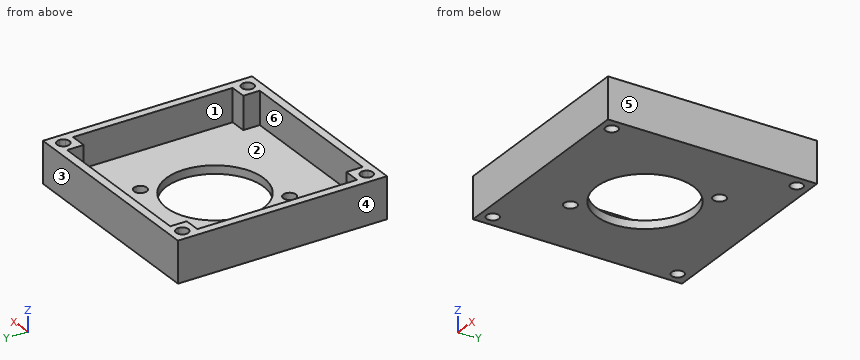
```python
from build123d import *
from build123d.topology import SkipClean

# Parameters (mm, degrees)
SKETCH3_W           = 50.8
SKETCH3_H           = 50.8
SKETCH3_R           = 11.8
SKETCH3_R_2         = 1.55
BOSS_EXTRUDE5_DEPTH = 2
SKETCH1_W           = 2
SKETCH1_H           = 38.8
SKETCH1_W_2         = 38.8
SKETCH1_H_2         = 2
BOSS_EXTRUDE6_DEPTH = 10
SKETCH7_R           = 1.5
CUT_EXTRUDE2_DEPTH  = 37.80108694


with BuildPart() as part:
    # Sketch3 → Boss-Extrude5 (new body)
    with BuildSketch(Plane.XY):
        Rectangle(SKETCH3_W, SKETCH3_H)
        Circle(SKETCH3_R, mode=Mode.SUBTRACT)
        with Locations((-9.5, -12)):
            Circle(SKETCH3_R_2, mode=Mode.SUBTRACT)
        with Locations((9.5, 12)):
            Circle(SKETCH3_R_2, mode=Mode.SUBTRACT)
    extrude(amount=BOSS_EXTRUDE5_DEPTH)

    # Sketch1 → Boss-Extrude6 (add)
    with BuildSketch(Plane.XY):
        with Locations((24.4, 0)):
            Rectangle(SKETCH1_W, SKETCH1_H)
        with BuildLine():
            Line((21.281966011, -23.4), (19.4, -23.4))
            Line((19.4, -23.4), (19.4, -25.4))
            Line((19.4, -25.4), (25.4, -25.4))
            Line((25.4, -25.4), (25.4, -19.4))
            Line((25.4, -19.4), (23.4, -19.4))
            Line((23.4, -19.4), (23.4, -21.281966011))
            ThreePointArc((23.4, -21.281966011), (23.769306394, -21.787627564), (23.9, -22.4))
            ThreePointArc((23.9, -22.4), (22.935233135, -23.801258538), (21.281966011, -23.4))
        make_face()
        with BuildLine():
            Line((19.4, -19.4), (19.4, -23.4))
            Line((19.4, -23.4), (21.281966011, -23.4))
            ThreePointArc((21.281966011, -23.4), (21.339339828, -21.339339828), (23.4, -21.281966011))
            Line((23.4, -21.281966011), (23.4, -19.4))
            Line((23.4, -19.4), (19.4, -19.4))
        make_face()
        with Locations((0, -24.4)):
            Rectangle(SKETCH1_W_2, SKETCH1_H_2)
        with BuildLine():
            ThreePointArc((-20.9, -22.4), (-20.998741462, -22.935233135), (-21.281966011, -23.4))
            Line((-21.281966011, -23.4), (-19.4, -23.4))
            Line((-19.4, -23.4), (-19.4, -19.4))
            Line((-19.4, -19.4), (-23.4, -19.4))
            Line((-23.4, -19.4), (-23.4, -21.281966011))
            ThreePointArc((-23.4, -21.281966011), (-21.787627564, -21.030693606), (-20.9, -22.4))
        make_face()
        with BuildLine():
            Line((-19.4, -23.4), (-21.281966011, -23.4))
            ThreePointArc((-21.281966011, -23.4), (-23.460660172, -23.460660172), (-23.4, -21.281966011))
            Line((-23.4, -21.281966011), (-23.4, -19.4))
            Line((-23.4, -19.4), (-25.4, -19.4))
            Line((-25.4, -19.4), (-25.4, -25.4))
            Line((-25.4, -25.4), (-19.4, -25.4))
            Line((-19.4, -25.4), (-19.4, -23.4))
        make_face()
        with Locations((-24.4, 0)):
            Rectangle(SKETCH1_W, SKETCH1_H)
        with BuildLine():
            Line((-25.4, 19.4), (-23.4, 19.4))
            Line((-23.4, 19.4), (-23.4, 21.281966011))
            ThreePointArc((-23.4, 21.281966011), (-23.460660172, 23.460660172), (-21.281966011, 23.4))
            Line((-21.281966011, 23.4), (-19.4, 23.4))
            Line((-19.4, 23.4), (-19.4, 25.4))
            Line((-19.4, 25.4), (-25.4, 25.4))
            Line((-25.4, 25.4), (-25.4, 19.4))
        make_face()
        with BuildLine():
            Line((-23.4, 21.281966011), (-23.4, 19.4))
            Line((-23.4, 19.4), (-19.4, 19.4))
            Line((-19.4, 19.4), (-19.4, 23.4))
            Line((-19.4, 23.4), (-21.281966011, 23.4))
            ThreePointArc((-21.281966011, 23.4), (-20.998741462, 22.935233135), (-20.9, 22.4))
            ThreePointArc((-20.9, 22.4), (-21.787627564, 21.030693606), (-23.4, 21.281966011))
        make_face()
        with Locations((0, 24.4)):
            Rectangle(SKETCH1_W_2, SKETCH1_H_2)
        with BuildLine():
            Line((23.4, 21.281966011), (23.4, 19.4))
            Line((23.4, 19.4), (25.4, 19.4))
            Line((25.4, 19.4), (25.4, 25.4))
            Line((25.4, 25.4), (19.4, 25.4))
            Line((19.4, 25.4), (19.4, 23.4))
            Line((19.4, 23.4), (21.281966011, 23.4))
            ThreePointArc((21.281966011, 23.4), (22.935233135, 23.801258538), (23.9, 22.4))
            ThreePointArc((23.9, 22.4), (23.769306394, 21.787627564), (23.4, 21.281966011))
        make_face()
        with BuildLine():
            Line((19.4, 19.4), (23.4, 19.4))
            Line((23.4, 19.4), (23.4, 21.281966011))
            ThreePointArc((23.4, 21.281966011), (21.339339828, 21.339339828), (21.281966011, 23.4))
            Line((21.281966011, 23.4), (19.4, 23.4))
            Line((19.4, 23.4), (19.4, 19.4))
        make_face()
    extrude(amount=BOSS_EXTRUDE6_DEPTH)

    # Sketch7 → Cut-Extrude2 (cut, through all)
    with SkipClean():  # the faces are left unmerged after this step: merging them gives an invalid solid
        with BuildSketch(Plane.XY.offset(2)):
            with Locations((-22.4, 22.4)):
                Circle(SKETCH7_R)
            with Locations(Location((22.4, 22.4, 0), (0, 0, 180))):
                Circle(SKETCH7_R)
            with Locations((22.4, -22.529256464)):
                Circle(SKETCH7_R)
            with Locations(Location((-22.4, -22.529256464, 0), (0, 0, 2.46938104))):
                Circle(SKETCH7_R)
        extrude(amount=-CUT_EXTRUDE2_DEPTH, mode=Mode.SUBTRACT)


solid = part.part
```
Could you check a few things on this model? Use its own coordinates, in mm. Face numbers are marked on the shaded views. A direction names the side the tool comes from. Give positions to 0.01 mm unless a question says otherwise; leave off trailing zeros. Write each loop counter-clockwise with the first axis right and the second up, starting at its lowest first coordinate (ties: lowest second). Pieces come first, ordered by that corner, then holes. Notation, with made-up numbers: (46.5, 22.25) - (56.5, 22.25) arc R29 cw to (56.5, 51.25) - close; hole circle Ø9 at (-18, 49.5). An arc over 180 degrees is marked (long way). One line per item, written item: value. Start each with the question number.
Item 1: Please list where these lines run through material, in increasing order: line 1 (Y direction, x = -22.4, z = 1.45); line 2 (X direction, y = 22.4, z = 1.05); line 3 (Y direction, x = 0, z = 0.5). Write a range as from..to.
Item 2: Imagine slicing it at A-A, the plane x = 22.4. List the corners of the cut face in (y, z) for me.
Item 3: Imagine slicing it at B-B, the plane z = 6.5. List the corners of the cut face in (x, y) for me.
Item 4: If we mould it in two halves opening along X, with no side actions, what happens to the marked faces 1, 2, 3 and 4? For each: +X half, -X half, draft (parallel to the pull), parting line (faces both ways), or undercut.
Item 5: Which directions (+Z, -Z, +X, -X, +Y, -Y) give clear straight access to the entire face, cutting with the end or side of a thin tool? Please do the marked faces 5 and 6.
Item 6: Imagine slicing it at C-C, the plane y = -4. List the corners of the cut face in (x, z) for me.
Item 7: Imagine slicing it at D-D, the plane z = 1. List the corners of the cut face in (x, y) for me, and give its area (3 significant figures).
Geometry says:
1. line 1: -25.4..-24.03, -21.03..20.9, 23.9..25.4
1. line 2: -25.4..-23.9, -20.9..20.9, 23.9..25.4
1. line 3: -25.4..-11.8, 11.8..25.4
2. outline: (-25.4, 0) - (-24.03, 0) - (-24.03, 2) - (-23.9, 2) - (-23.9, 10) - (-25.4, 10) - close; (-21.03, 0) - (20.9, 0) - (20.9, 10) - (19.4, 10) - (19.4, 2) - (-19.4, 2) - (-19.4, 10) - (-20.9, 10) - (-20.9, 2) - (-21.03, 2) - close; (23.9, 0) - (25.4, 0) - (25.4, 10) - (23.9, 10) - close
3. outline: (-25.4, -25.4) - (25.4, -25.4) - (25.4, 25.4) - (-25.4, 25.4) - close; hole circle Ø3 at (-22.4, -22.4); hole circle Ø3 at (-22.4, 22.4); hole (-23.4, -19.4) - (-19.4, -19.4) - (-19.4, -23.4) - (19.4, -23.4) - (19.4, -19.4) - (23.4, -19.4) - (23.4, 19.4) - (19.4, 19.4) - (19.4, 23.4) - (-19.4, 23.4) - (-19.4, 19.4) - (-23.4, 19.4) - close; hole circle Ø3 at (22.4, -22.4); hole circle Ø3 at (22.4, 22.4)
4. face 1: undercut
4. face 2: undercut
4. face 3: draft
4. face 4: -X half
5. face 5: +Z, -Z, +X, +Y, -Y
5. face 6: +Z
6. outline: (-25.4, 0) - (-11.1, 0) - (-11.1, 2) - (-23.4, 2) - (-23.4, 10) - (-25.4, 10) - close; (11.1, 0) - (25.4, 0) - (25.4, 10) - (23.4, 10) - (23.4, 2) - (11.1, 2) - close
7. outline: (-25.4, -25.4) - (25.4, -25.4) - (25.4, 25.4) - (-25.4, 25.4) - close; hole circle Ø3 at (-22.4, -22.53); hole circle Ø3 at (-22.4, 22.4); hole circle Ø23.6 at (0, 0); hole circle Ø3.1 at (-9.5, -12); hole circle Ø3.1 at (9.5, 12); hole circle Ø3 at (22.4, -22.53); hole circle Ø3 at (22.4, 22.4)
7. area: 2,100 mm^2
